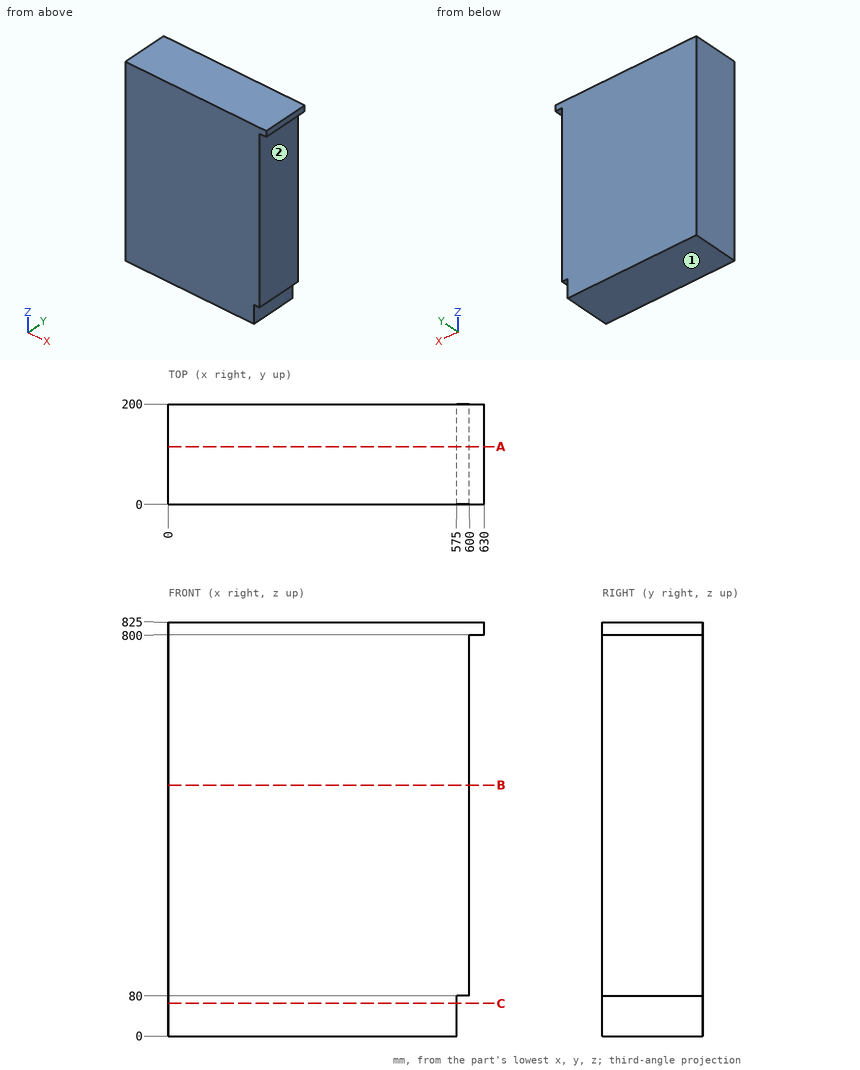
The drawing under review shows one solid part. Ordinate dimensions are in mm from its lowest x, y, z. A direction names the side the tool comes from. Give positions to 0.01 mm unless a question says otherwise; leave off trailing zeros. Write each loop counter-clockwise with the first axis right and the second up, starting at its lowest first coordinate (ties: lowest second). Pieces come first, ordered by that corner, then holes. Notation, with made-up numbers: M -9.5,40.25 L 14.5,40.25 A20 ccw 14.5,66.25 Z; hole C 1,-40 d8. An arc over 180 degrees is marked long. Write each question's results on one line, items separated by ' | '. Start each with the question number.
1. We need section A-A (y = 115). Write out the cut boundary in (x, z).
2. For the marked faces 1 and 2, list the 3-axis set-ups (+Z, -Z, +X, -X, +Y, -Y) from which the entire face can be reached by the end or side of a thin tool; tool diameter is ignored.
3. For probe 1 along X at (y, z) = (53.5, 266.5); probe 2 along X at (y, z) = (76.5, 49), list the stretches that pass through material, from the lowest coordinate up. Write a range as [from, to].
4. We need section B-B (z = 500.5). Write out the cut boundary in (x, y).
5. We need section C-C (z = 65). Write out the cut boundary in (x, y), and give its area (3 significant figures).
6. Insertion check: pin 1 Ø10 at (y, z) = (146.5, 234.5) entering from +X; pin 2 Ø12.5 at (x, y) = (588.5, 146) entering from -Z; pin 3 Ø24 at (y, z) = (51, 41.5) entering from +X. Each pin has a flat end and moves straight along its axis. Give the tip position at first contact, or say it passes through.
Results found:
1) outline: M 0,0 L 575,0 L 575,80 L 600,80 L 600,800 L 630,800 L 630,825 L 0,825 Z
2) face 1: -Z, +X, -X, +Y, -Y | face 2: -Z, +X, +Y, -Y
3) probe 1: x = [0, 600] | probe 2: x = [0, 575]
4) outline: M 0,0 L 600,0 L 600,200 L 0,200 Z
5) outline: M 0,0 L 575,0 L 575,200 L 0,200 Z | area: 115,000 mm^2
6) pin 1: stops at x = 600 | pin 2: stops at z = 80 | pin 3: stops at x = 575
